Read the model definition and answer for the solid it produces. Units are mm, in the model's axes. A direction names the side the tool comes from. Round coordinates to 2 decimals unless told otherwise and drop trailing zeros. Write each loop counter-clockwise with the first axis right and the second up, starting at its lowest first coordinate (ties: lowest second). Pieces come first, ordered by that corner, then holes. Notation, with made-up numbers: (5.5, 63) -> (22.5, 63) arc R37 ccw to (22.5, 102) -> close; hole circle Ø6 at (-12.75, 68). An arc over 180 degrees is marked (long way). Return JSON: item names as keys, results as strings. Group by question number.
(1) A cutting plane is placed at C-C on z = 3.5. Give the vertices of the cut face in (x, y).
(2) Given pin 1 (1 mm diameter, centred on x = 2.5, z = 12, fed in from +Y); pin 2 (1.5 mm diameter, centred on x = 4.5, z = 13, fed in from +Y); pin 3 (2 mm diameter, centred on x = -4, y = -2, fed in from -Z); pin 4 (0.6 mm diameter, centred on x = -4.5, z = 11, fed in from +Y), each flat-ended and moving along its own axis, determine where each tip first touches the part or whether it passes through.
(3) The mould has two halves that part along Z. Classify faces 5 (the flat face through (0, -3, 18.5)), 6 (the flat face through (0, -3, 0)), 7 (the cylindrical face through (-2.351, 4.413, 12.176)): released by +Z, released by -Z, zero draft, split by the parting line, or undercut.
(4) For faces 1 (the cylindrical face through (-0.42, -4.23, 12.18)), 2 (the flat face through (1.5, -4.6, 17.5)), 3 (the cylindrical face through (4.783, -1.458, 12.176)), 4 (the cylindrical face through (1.458, 4.783, 12.176)), determine the directions among +Z, -Z, +X, -X, +Y, -Y from which every point of the face is accessible in a straight line to the end or side of a thin tool.
(5) A cutting plane is placed at A-A on y = -5.75. Give the vertices of the cut face in (x, z).
(6) A cutting plane is placed at B-B on x = 0.25. Give the vertices of the cut face in (y, z), then the cut area to 3 significant figures.
(7) Straight lines are drawn through the part: line 1 (Y direction, x = 0, z = 5); line 2 (X direction, y = -4.5, z = 13.5); line 3 (Z direction, x = -5.5, y = -4). For each, find the intervals that lie inside material, in ascending order.
```python
from build123d import *

# Parameters (mm, degrees)
F0_R     = 7
F1_DEPTH = 7
F3_DEPTH = 10.5
F4_R     = 7
F5_DEPTH = 1
F6_R     = 2.5
F7_DEPTH = 18.501
F8_R     = 1.5
F9_DEPTH = 25


with BuildPart() as f1:
    # F0 (on Top) → F1 (new body)
    with BuildSketch(Plane.XY):
        Circle(F0_R)
    extrude(amount=F1_DEPTH)

    # F2 (on face) → F3 (join)
    with BuildSketch(Plane.XY.offset(7)):
        with BuildLine():
            ThreePointArc((0.829134, 4.168337), (0.416573, 4.229535), (0, 4.25))
            Line((0, 4.25), (0, 5))
            ThreePointArc((0, 5), (-0.490086, 4.975924), (-0.975452, 4.903926))
            Line((-0.975452, 4.903926), (-0.829134, 4.168337))
            ThreePointArc((-0.829134, 4.168337), (-1.23371, 4.066996), (-1.626405, 3.926488))
            Line((-1.626405, 3.926488), (-1.913417, 4.619398))
            ThreePointArc((-1.913417, 4.619398), (-2.356984, 4.409606), (-2.777851, 4.157348))
            Line((-2.777851, 4.157348), (-2.361173, 3.533746))
            ThreePointArc((-2.361173, 3.533746), (-2.696171, 3.285294), (-3.005204, 3.005204))
            Line((-3.005204, 3.005204), (-3.535534, 3.535534))
            ThreePointArc((-3.535534, 3.535534), (-3.865052, 3.171966), (-4.157348, 2.777851))
            Line((-4.157348, 2.777851), (-3.533746, 2.361173))
            ThreePointArc((-3.533746, 2.361173), (-3.748165, 2.003436), (-3.926488, 1.626405))
            Line((-3.926488, 1.626405), (-4.619398, 1.913417))
            ThreePointArc((-4.619398, 1.913417), (-4.784702, 1.451423), (-4.903926, 0.975452))
            Line((-4.903926, 0.975452), (-4.168337, 0.829134))
            ThreePointArc((-4.168337, 0.829134), (-4.229535, 0.416573), (-4.25, 0))
            Line((-4.25, 0), (-5, 0))
            ThreePointArc((-5, 0), (-4.975924, -0.490086), (-4.903926, -0.975452))
            Line((-4.903926, -0.975452), (-4.168337, -0.829134))
            ThreePointArc((-4.168337, -0.829134), (-4.066996, -1.23371), (-3.926488, -1.626405))
            Line((-3.926488, -1.626405), (-4.619398, -1.913417))
            ThreePointArc((-4.619398, -1.913417), (-4.409606, -2.356984), (-4.157348, -2.777851))
            Line((-4.157348, -2.777851), (-3.533746, -2.361173))
            ThreePointArc((-3.533746, -2.361173), (-3.285294, -2.696171), (-3.005204, -3.005204))
            Line((-3.005204, -3.005204), (-3.535534, -3.535534))
            ThreePointArc((-3.535534, -3.535534), (-3.171966, -3.865052), (-2.777851, -4.157348))
            Line((-2.777851, -4.157348), (-2.361173, -3.533746))
            ThreePointArc((-2.361173, -3.533746), (-2.003436, -3.748165), (-1.626405, -3.926488))
            Line((-1.626405, -3.926488), (-1.913417, -4.619398))
            ThreePointArc((-1.913417, -4.619398), (-1.451423, -4.784702), (-0.975452, -4.903926))
            Line((-0.975452, -4.903926), (-0.829134, -4.168337))
            ThreePointArc((-0.829134, -4.168337), (-0.416573, -4.229535), (0, -4.25))
            Line((0, -4.25), (0, -5))
            ThreePointArc((0, -5), (0.490086, -4.975924), (0.975452, -4.903926))
            Line((0.975452, -4.903926), (0.829134, -4.168337))
            ThreePointArc((0.829134, -4.168337), (1.23371, -4.066996), (1.626405, -3.926488))
            Line((1.626405, -3.926488), (1.913417, -4.619398))
            ThreePointArc((1.913417, -4.619398), (2.356984, -4.409606), (2.777851, -4.157348))
            Line((2.777851, -4.157348), (2.361173, -3.533746))
            ThreePointArc((2.361173, -3.533746), (2.696171, -3.285294), (3.005204, -3.005204))
            Line((3.005204, -3.005204), (3.535534, -3.535534))
            ThreePointArc((3.535534, -3.535534), (3.865052, -3.171966), (4.157348, -2.777851))
            Line((4.157348, -2.777851), (3.533746, -2.361173))
            ThreePointArc((3.533746, -2.361173), (3.748165, -2.003436), (3.926488, -1.626405))
            Line((3.926488, -1.626405), (4.619398, -1.913417))
            ThreePointArc((4.619398, -1.913417), (4.784702, -1.451423), (4.903926, -0.975452))
            Line((4.903926, -0.975452), (4.168337, -0.829134))
            ThreePointArc((4.168337, -0.829134), (4.229535, -0.416573), (4.25, 0))
            Line((4.25, 0), (5, 0))
            ThreePointArc((5, 0), (4.975924, 0.490086), (4.903926, 0.975452))
            Line((4.903926, 0.975452), (4.168337, 0.829134))
            ThreePointArc((4.168337, 0.829134), (4.066996, 1.23371), (3.926488, 1.626405))
            Line((3.926488, 1.626405), (4.619398, 1.913417))
            ThreePointArc((4.619398, 1.913417), (4.409606, 2.356984), (4.157348, 2.777851))
            Line((4.157348, 2.777851), (3.533746, 2.361173))
            ThreePointArc((3.533746, 2.361173), (3.285294, 2.696171), (3.005204, 3.005204))
            Line((3.005204, 3.005204), (3.535534, 3.535534))
            ThreePointArc((3.535534, 3.535534), (3.171966, 3.865052), (2.777851, 4.157348))
            Line((2.777851, 4.157348), (2.361173, 3.533746))
            ThreePointArc((2.361173, 3.533746), (2.003436, 3.748165), (1.626405, 3.926488))
            Line((1.626405, 3.926488), (1.913417, 4.619398))
            ThreePointArc((1.913417, 4.619398), (1.451423, 4.784702), (0.975452, 4.903926))
            Line((0.975452, 4.903926), (0.829134, 4.168337))
        make_face()
    extrude(amount=F3_DEPTH)

    # F4 (on face) → F5 (join)
    with BuildSketch(Plane.XY.offset(17.5)):
        Circle(F4_R)
    extrude(amount=F5_DEPTH)

    # F6 (on face) → F7 (cut, through all)
    with BuildSketch(Plane(origin=(0, 0, 0), x_dir=(1, 0, 0), z_dir=(0, 0, -1))):
        Circle(F6_R)
    extrude(amount=-F7_DEPTH, mode=Mode.SUBTRACT)

    # F8 (on Right) → F9 (cut)
    with BuildSketch(Plane.YZ):
        with Locations((0, 3.5)):
            Circle(F8_R)
    extrude(amount=-F9_DEPTH, mode=Mode.SUBTRACT)


solid = f1.part
```
Checks:
{
 "1": {"outline": "(-6.84, -1.5) arc R7 ccw (long way) to (-6.84, 1.5) -> (-2, 1.5) arc R2.5 cw (long way) to (-2, -1.5) -> close"},
 "2": {"pin 1": "stops at y = 4.16", "pin 2": "stops at y = 2.78", "pin 3": "stops at z = 0", "pin 4": "stops at y = 1.91"},
 "3": {"face 5": "released by +Z", "face 6": "released by -Z", "face 7": "undercut"},
 "4": {"face 1": "-Y", "face 2": "none", "face 3": "+X, -Y", "face 4": "+X, +Y"},
 "5": {"outline": "(-3.99, 0) -> (3.99, 0) -> (3.99, 7) -> (-3.99, 7) -> close; (-3.99, 17.5) -> (3.99, 17.5) -> (3.99, 18.5) -> (-3.99, 18.5) -> close"},
 "6": {"outline": "(-7, 0) -> (-2.49, 0) -> (-2.49, 18.5) -> (-7, 18.5) -> (-7, 17.5) -> (-4.99, 17.5) -> (-4.99, 7) -> (-7, 7) -> close; (2.49, 0) -> (7, 0) -> (7, 7) -> (4.24, 7) -> (4.24, 17.5) -> (7, 17.5) -> (7, 18.5) -> (2.49, 18.5) -> close", "area": "117 mm^2"},
 "7": {"line 1": "y = -7 to -2.5, 2.5 to 7", "line 2": "x = -1.86 to -0.9, 0 to 0.9, 1.86 to 2.18", "line 3": "z = 0 to 7, 17.5 to 18.5"}
}
